from build123d import *

# Parameters (mm, degrees)
EXTRUDE_1_DEPTH       = 23
SKETCH_2_R            = 11.75
CUT_EXTRUDE_1_DEPTH   = 2
SKETCH_3_R            = 7.6
CUT_EXTRUDE_2_DEPTH   = 4
SKETCH_4_R            = 7.05
CUT_EXTRUDE_3_DEPTH   = 4
SKETCH_5_R            = 6.1
CUT_EXTRUDE_4_DEPTH   = 4
SKETCH_6_R            = 2.6
CUT_EXTRUDE_5_DEPTH   = 9
SKETCH_7_R            = 2.95
CUT_EXTRUDE_6_DEPTH   = 1.1
SKETCH_8_W            = 50.7
SKETCH_8_H            = 19.2
CUT_EXTRUDE_7_DEPTH   = 8.1
SKETCH_9_W            = 60.5
SKETCH_9_H            = 23
CUT_EXTRUDE_8_DEPTH   = 14.9
CUT_EXTRUDE_9_REACH   = 94.5
SKETCH_10_W           = 8
SKETCH_10_H           = 10
CUT_EXTRUDE_1_2_DEPTH = 2.1
SKETCH_13_W           = 12.2
SKETCH_13_H           = 12.2
CUT_EXTRUDE_11_DEPTH  = 1.5
CUT_EXTRUDE_14_REACH  = 3
SKETCH_16_R           = 3.5
SKETCH_14_W           = 2.7
SKETCH_14_H           = 5.5
CUT_EXTRUDE_12_DEPTH  = 12
SKETCH_15_W           = 2.9
SKETCH_15_H           = 5.7
CUT_EXTRUDE_13_DEPTH  = 5.6
FILLET_1_R            = 0.5


with BuildPart() as part:
    # Эскиз1 → Бобышка-Вытянуть1 (new body)
    with BuildSketch(Plane.XY):
        with BuildLine():
            Line((39.25, -14), (-39.25, -14))
            ThreePointArc((-39.25, -14), (-53.25, 0), (-39.25, 14))
            Line((-39.25, 14), (39.25, 14))
            Line((39.25, 14), (39.25, -14))
        make_face()
    extrude(amount=EXTRUDE_1_DEPTH)

    # Эскиз2 → Cut-Extrude 1 (cut)
    with BuildSketch(Plane.XY.offset(23)):
        with Locations((-39.25, 0)):
            Circle(SKETCH_2_R)
    extrude(amount=-CUT_EXTRUDE_1_DEPTH, mode=Mode.SUBTRACT)

    # Эскиз3 → Вырез-Вытянуть2 (cut)
    with BuildSketch(Plane.XY.offset(21)):
        with Locations((-39.25, 0)):
            Circle(SKETCH_3_R)
    extrude(amount=-CUT_EXTRUDE_2_DEPTH, mode=Mode.SUBTRACT)

    # Эскиз4 → Вырез-Вытянуть3 (cut)
    with BuildSketch(Plane.XY.offset(17)):
        with Locations((-39.25, 0)):
            Circle(SKETCH_4_R)
    extrude(amount=-CUT_EXTRUDE_3_DEPTH, mode=Mode.SUBTRACT)

    # Эскиз5 → Вырез-Вытянуть4 (cut)
    with BuildSketch(Plane.XY.offset(13)):
        with Locations((-39.25, 0)):
            Circle(SKETCH_5_R)
    extrude(amount=-CUT_EXTRUDE_4_DEPTH, mode=Mode.SUBTRACT)

    # Эскиз6 → Вырез-Вытянуть5 (cut)
    with BuildSketch(Plane.XY.offset(9)):
        with Locations((-39.25, 0)):
            Circle(SKETCH_6_R)
    extrude(amount=-CUT_EXTRUDE_5_DEPTH, mode=Mode.SUBTRACT)

    # Эскиз7 → Вырез-Вытянуть6 (cut)
    with BuildSketch(Plane(origin=(0, 0, 0), x_dir=(-1, 0, 0), z_dir=(0, 0, -1))):
        with Locations((39.25, 0)):
            Circle(SKETCH_7_R)
    extrude(amount=-CUT_EXTRUDE_6_DEPTH, mode=Mode.SUBTRACT)

    # Эскиз8 → Вырез-Вытянуть7 (cut)
    with BuildSketch(Plane.XY.offset(23)):
        with Locations((9.5, 0)):
            Rectangle(SKETCH_8_W, SKETCH_8_H)
    extrude(amount=-CUT_EXTRUDE_7_DEPTH, mode=Mode.SUBTRACT)

    # Эскиз9 → Вырез-Вытянуть8 (cut)
    with BuildSketch(Plane(origin=(0, 0, 0), x_dir=(-1, 0, 0), z_dir=(0, 0, -1))):
        with Locations((-6.5, 0)):
            Rectangle(SKETCH_9_W, SKETCH_9_H)
    extrude(amount=-CUT_EXTRUDE_8_DEPTH, mode=Mode.SUBTRACT)

    # Эскиз10 → Вырез-Вытянуть9 (cut, up to next)
    with BuildSketch(Plane(origin=(39.25, 0, 0), x_dir=(0, 0, -1), z_dir=(1, 0, 0)), mode=Mode.PRIVATE) as cut_extrude_9_sk1:
        with Locations((-10, 0)):
            Rectangle(SKETCH_10_W, SKETCH_10_H)
    cut_extrude_9_tool1 = extrude(cut_extrude_9_sk1.sketch, amount=-CUT_EXTRUDE_9_REACH, mode=Mode.PRIVATE) & part.part
    add(cut_extrude_9_tool1.solids().sort_by_distance((39.25, 0, 10))[0], mode=Mode.SUBTRACT)

    # Эскиз11 → Cut-Extrude 1 2 (cut)
    with BuildSketch(Plane(origin=(0, 0, 0), x_dir=(-1, 0, 0), z_dir=(0, 0, -1))):
        with BuildLine():
            Line((39.25, 15), (-40.25, 15))
            Line((-40.25, 15), (-40.25, -15))
            Line((-40.25, -15), (39.25, -15))
            ThreePointArc((39.25, -15), (54.25, 0), (39.25, 15))
        make_face()
        with BuildLine():
            Line((39.25, 13), (-38.25, 13))
            Line((-38.25, 13), (-38.25, -13))
            Line((-38.25, -13), (39.25, -13))
            ThreePointArc((39.25, -13), (52.25, 0), (39.25, 13))
        make_face(mode=Mode.SUBTRACT)
    extrude(amount=-CUT_EXTRUDE_1_2_DEPTH, mode=Mode.SUBTRACT)

    # Эскиз13 → Вырез-Вытянуть11 (cut)
    with BuildSketch(Plane(origin=(0, -11.5, 0), x_dir=(1, 0, 0), z_dir=(0, 1, 0))):
        with Locations((3.25, -8.8)):
            Rectangle(SKETCH_13_W, SKETCH_13_H)
    extrude(amount=-CUT_EXTRUDE_11_DEPTH, mode=Mode.SUBTRACT)

    # Эскиз16 → Вырез-Вытянуть14 (cut, up to next)
    with BuildSketch(Plane(origin=(0, -13, 0), x_dir=(1, 0, 0), z_dir=(0, 1, 0)), mode=Mode.PRIVATE) as cut_extrude_14_sk1:
        with Locations((3.25, -8.8)):
            Circle(SKETCH_16_R)
    cut_extrude_14_tool1 = extrude(cut_extrude_14_sk1.sketch, amount=-CUT_EXTRUDE_14_REACH, mode=Mode.PRIVATE) & part.part
    add(cut_extrude_14_tool1.solids().sort_by_distance((3.25, -13, 8.8))[0], mode=Mode.SUBTRACT)

    # Эскиз14 → Вырез-Вытянуть12 (cut)
    with BuildSketch(Plane(origin=(0, 0, 14.9), x_dir=(-1, 0, 0), z_dir=(0, 0, -1))):
        with Locations((22.4, 0)):
            Rectangle(SKETCH_14_W, SKETCH_14_H)
    extrude(amount=-CUT_EXTRUDE_12_DEPTH, mode=Mode.SUBTRACT)

    # Эскиз15 → Вырез-Вытянуть13 (cut)
    with BuildSketch(Plane.XY.offset(23)):
        with Locations((-22.4, 0)):
            Rectangle(SKETCH_15_W, SKETCH_15_H)
    extrude(amount=-CUT_EXTRUDE_13_DEPTH, mode=Mode.SUBTRACT)

    # Скругление1
    fillet_1_edges = [part.edges().sort_by_distance(p)[0] for p in [
        (39.25, 0, 23),
        (0, 14, 23),
        (-53.25, 0, 23),
        (0, -14, 23),
        (39.25, 14, 12.55),
        (39.25, -14, 12.55),
    ]]
    fillet(fillet_1_edges, radius=FILLET_1_R)


solid = part.part
Work out the finished part from the listing and answer in its coordinate system (mm). A direction names the side the tool comes from. Round coordinates to 2 decimals unless told otherwise and drop trailing zeros. Write each loop counter-clockwise with the first axis right and the second up, starting at its lowest first coordinate (ties: lowest second). Pieces come first, ordered by that corner, then holes. Notation, with made-up numbers: (86, 12.5) -> (139, 12.5) arc R21 cw to (139, 50.5) -> close; hole circle Ø5 at (71, -36.75). An arc over 180 degrees is marked (long way). Answer as CSV lines item,"result". Start each with the question number.
(1) The part is cut by section C-C, the plane x = 3.25. Give the vertices of the cut face in (y, z).
(2) The part is cut by section A-A, the plane x = 27. Give the vertices of the cut face in (y, z), then the cut area to 3 significant figures.
(3) Find the intervals of material crossed by probe 1 along Y at (x, z) = (-21, 5.5); probe 2 along Y at (x, z) = (-39.25, 14.25); probe 3 along X at (y, z) = (-11.75, 3.5), in increasing order.
(4) The part is cut by section B-B, the plane z = 18.5. Give the vertices of the cut face in (x, y).
(5) The part is cut by section D-D, the plane z = 10.5. Give the vertices of the cut face in (x, y).
(6) The mould has two halves that part along Z. Classify faces 1 (the flat face through (7, 11.5, 7)), 2 (the flat face through (5.9, -13, 11.4)), 3 (the flat face through (-39, -3, 9)): +Z half, -Z half, draft (parallel to the pull), parting line (faces both ways), or undercut.
(7) Each of these flat-tipped pins is pushed along its axis until it touches: pin 1 (3 mm diameter, centred on x = -43, z = 4, fed in from -Y); pin 2 (4.5 mm diameter, centred on x = -36, y = 3, fed in from +Z); pin 3 (5 mm diameter, centred on x = -43, z = 18, fed in from +Y). Where does it stop, or does it pass through?
(8) A tool of negligible diameter and unlimited length cuts with its end or side. For faces 4 (the flat face through (38, -5, 10)), 5 (the flat face through (-23.85, 0, 20)), 6 (the flat face through (-2.85, -12, 9)), from which of +Z, -Z, +X, -X, +Y, -Y can it reach the whole face along a straight path? Write none if from no direction.
Output values:
1,outline,"(-14, 2.1) -> (-13, 2.1) -> (-13, 0) -> (-11.5, 0) -> (-11.5, 2.7) -> (-13, 2.7) -> (-13, 5.3) -> (-14, 5.3) -> close; (-14, 12.3) -> (-13, 12.3) -> (-13, 14.9) -> (-9.6, 14.9) -> (-9.6, 23) -> (-13.5, 23) arc R0.5 ccw to (-14, 22.5) -> close; (9.6, 14.9) -> (11.5, 14.9) -> (11.5, 0) -> (13, 0) -> (13, 2.1) -> (14, 2.1) -> (14, 22.5) arc R0.5 ccw to (13.5, 23) -> (9.6, 23) -> close"
2,outline,"(-14, 2.1) -> (-13, 2.1) -> (-13, 0) -> (-11.5, 0) -> (-11.5, 14.9) -> (-9.6, 14.9) -> (-9.6, 23) -> (-13.5, 23) arc R0.5 ccw to (-14, 22.5) -> close; (9.6, 14.9) -> (11.5, 14.9) -> (11.5, 0) -> (13, 0) -> (13, 2.1) -> (14, 2.1) -> (14, 22.5) arc R0.5 ccw to (13.5, 23) -> (9.6, 23) -> close"
2,area,"141 mm²"
3,probe 1,"y = -14 to -11.5, 11.5 to 14"
3,probe 2,"y = -14 to -7.05, 7.05 to 14"
3,probe 3,"x = -46.86 to -2.85, 9.35 to 39.25"
4,outline,"(-39.25, -14) -> (38.75, -14) arc R0.5 ccw to (39.25, -13.5) -> (39.25, 13.5) arc R0.5 ccw to (38.75, 14) -> (-39.25, 14) arc R14 ccw to start; hole circle Ø15.2 at (-39.25, 0); hole (-23.85, -2.85) -> (-20.95, -2.85) -> (-20.95, 2.85) -> (-23.85, 2.85) -> close; hole (-15.85, -9.6) -> (34.85, -9.6) -> (34.85, 9.6) -> (-15.85, 9.6) -> close"
5,outline,"(-39.25, -14) -> (0.19, -14) -> (0.19, -13) -> (-2.85, -13) -> (-2.85, -11.5) -> (-23.75, -11.5) -> (-23.75, 11.5) -> (36.75, 11.5) -> (36.75, 5) -> (39.25, 5) -> (39.25, 13.5) arc R0.5 ccw to (38.75, 14) -> (-39.25, 14) arc R14 ccw to start; (6.31, -14) -> (38.75, -14) arc R0.5 ccw to (39.25, -13.5) -> (39.25, -5) -> (36.75, -5) -> (36.75, -11.5) -> (9.35, -11.5) -> (9.35, -13) -> (6.31, -13) -> close; hole circle Ø12.2 at (-39.25, 0)"
6,face 1,"draft"
6,face 2,"undercut"
6,face 3,"+Z half"
7,pin 1,"stops at y = -13.82"
7,pin 2,"stops at z = 13"
7,pin 3,"stops at y = 13.94"
8,face 4,"+X"
8,face 5,"+Z"
8,face 6,"none"
